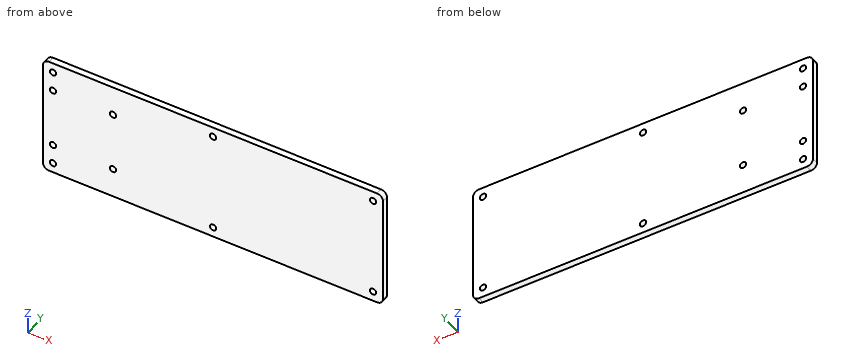
from build123d import *

# Parameters (mm, degrees)
SKETCH1_W           = 170
SKETCH1_H           = 60
BOSS_EXTRUDE1_DEPTH = 3.175
SKETCH2_R           = 1.6
CUT_EXTRUDE1_DEPTH  = 91.1946818
SKETCH3_R           = 1.6
CUT_EXTRUDE2_DEPTH  = 91.1946818
FILLET1_R           = 3


with BuildPart() as part:
    # Sketch1 → Boss-Extrude1 (new body)
    with BuildSketch(Plane(origin=(0, 0, 0), x_dir=(1, 0, 0), z_dir=(0, 1, 0))):
        Rectangle(SKETCH1_W, SKETCH1_H)
    extrude(amount=BOSS_EXTRUDE1_DEPTH)

    # Sketch2 → Cut-Extrude1 (cut, through all)
    with BuildSketch(Plane(origin=(0, 3.175, 0), x_dir=(1, 0, 0), z_dir=(0, 1, 0))):
        with Locations(Location((-80, -25, 0), (0, 0, 270))):
            Circle(SKETCH2_R)
        with Locations(Location((-80, 25, 0), (0, 0, 90))):
            Circle(SKETCH2_R)
        with Locations(Location((80, 25, 0), (0, 0, 270))):
            Circle(SKETCH2_R)
        with Locations(Location((80, -25, 0), (0, 0, 90))):
            Circle(SKETCH2_R)
        with Locations(Location((0, -25, 0), (0, 0, 270))):
            Circle(SKETCH2_R)
        with Locations(Location((0, 25, 0), (0, 0, 90))):
            Circle(SKETCH2_R)
    extrude(amount=-CUT_EXTRUDE1_DEPTH, mode=Mode.SUBTRACT)

    # Sketch3 → Cut-Extrude2 (cut, through all)
    with BuildSketch(Plane(origin=(0, 3.175, 0), x_dir=(1, 0, 0), z_dir=(0, 1, 0))):
        with Locations(Location((-80, -15, 0), (0, 0, 270))):
            Circle(SKETCH3_R)
        with Locations(Location((-80, 15, 0), (0, 0, 90))):
            Circle(SKETCH3_R)
        with Locations(Location((-50, 15, 0), (0, 0, 270))):
            Circle(SKETCH3_R)
        with Locations(Location((-50, -15, 0), (0, 0, 90))):
            Circle(SKETCH3_R)
    extrude(amount=-CUT_EXTRUDE2_DEPTH, mode=Mode.SUBTRACT)

    # Fillet1
    fillet1_edges = [part.edges().sort_by_distance(p)[0] for p in [
        (85, 1.5875, 30),
        (-85, 1.5875, 30),
        (-85, 1.5875, -30),
        (85, 1.5875, -30),
    ]]
    fillet(fillet1_edges, radius=FILLET1_R)


solid = part.part
Can you work these out from the model? Positions are in its coordinate system, mm. Coordinates: 2 decimals unless noted, no trailing zeros. Loops run counter-clockwise (first coordinate to the right, second up) from the corner with the lowest first, then second, coordinate; pieces in that order, holes last. Notation, with made-up numbers: (68, -20.5) - (108, -20.5) arc R22 cw to (108, -9.5) - close; hole circle Ø4 at (37.5, 35). An arc over 180 degrees is marked (long way). Put each result on its own line as item: value. Start each with the question number.
Item 1: For pin 1 (3 mm diameter, centred on x = 80, z = -25, fed in from -Y), with a flat end and sliding along its axis, tell me the tip position at first contact or that it passes through.
Item 2: Suppose I cut it at A-A (x = -50). Please give me the cut outline in (y, z) (3 decimals), and give its area (3 significant figures).
Item 3: If I drill on line 1 along Z through (x, y) = (-80, 1); line 2 along X through (y, z) = (2.5, -25); line 3 along Z through (x, y) = (80, 0.85), over which ranges is the centre line in solid material (lowest first)?
Item 4: Suppose I cut it at D-D (x = -80). Please give me the cut outline in (y, z) (3 decimals).
Item 5: Suppose I cut it at C-C (z = -15). Please give me the cut outline in (x, y) (3 decimals).
Item 6: Suppose I cut it at B-B (z = -25). Please give me the cut outline in (x, y) (3 decimals).
Here are the results:
1. pin 1: through
2. outline: (0, -30) - (3.175, -30) - (3.175, -16.6) - (0, -16.6) - close; (0, -13.4) - (3.175, -13.4) - (3.175, 13.4) - (0, 13.4) - close; (0, 16.6) - (3.175, 16.6) - (3.175, 30) - (0, 30) - close
2. area: 170 mm²
3. line 1: -30 to -26.6, -23.4 to -16.6, -13.4 to 13.4, 16.6 to 23.4, 26.6 to 30
3. line 2: -85 to -81.6, -78.4 to -1.6, 1.6 to 78.4, 81.6 to 85
3. line 3: -30 to -26.6, -23.4 to 23.4, 26.6 to 30
4. outline: (0, -30) - (3.175, -30) - (3.175, -26.6) - (0, -26.6) - close; (0, -23.4) - (3.175, -23.4) - (3.175, -16.6) - (0, -16.6) - close; (0, -13.4) - (3.175, -13.4) - (3.175, 13.4) - (0, 13.4) - close; (0, 16.6) - (3.175, 16.6) - (3.175, 23.4) - (0, 23.4) - close; (0, 26.6) - (3.175, 26.6) - (3.175, 30) - (0, 30) - close
5. outline: (-85, 0) - (-81.6, 0) - (-81.6, 3.175) - (-85, 3.175) - close; (-78.4, 0) - (-51.6, 0) - (-51.6, 3.175) - (-78.4, 3.175) - close; (-48.4, 0) - (85, 0) - (85, 3.175) - (-48.4, 3.175) - close
6. outline: (-85, 0) - (-81.6, 0) - (-81.6, 3.175) - (-85, 3.175) - close; (-78.4, 0) - (-1.6, 0) - (-1.6, 3.175) - (-78.4, 3.175) - close; (1.6, 0) - (78.4, 0) - (78.4, 3.175) - (1.6, 3.175) - close; (81.6, 0) - (85, 0) - (85, 3.175) - (81.6, 3.175) - close
